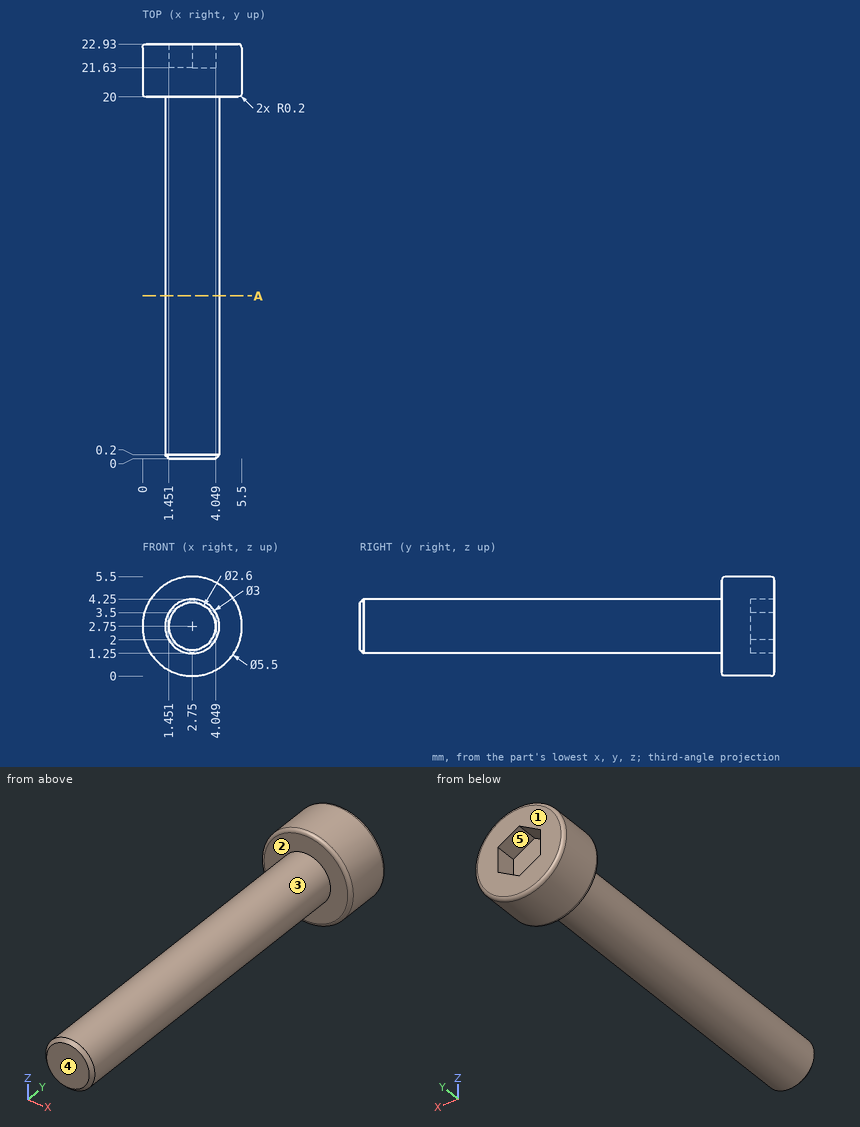
Verification items for this drawing (mm, ordinates from the low corner). A direction names the side the tool comes from. Round coordinates to 2 decimals unless told otherwise and drop trailing zeros. Order: outer loops, then holes, each group sorted by start corner. A loop starts at its lowest first (then second) coordinate and runs counter-clockwise, first axis right, second up.
1) Cross-section at A-A, the plane y = 9. Record the cut outline in (x, z), plus the area to 3 significant figures.
Geometry says:
outline: circle Ø3 at (2.75, 2.75)
area: 7.07 mm2
2) Tool access check on the marked faces 1 and 2. Record the directions out of +Z, -Z, +X, -X, +Y, -Y that give a thin tool (end or side, any length) a straight path to the whole face; none if there is none.
Geometry says:
face 1: +Z, -Z, +X, -X, +Y
face 2: -Y
3) Material ranges on line 1 (Y direction, x = 4.45, z = 1.4); line 2 (Y direction, x = 2.2, z = 2.1); line 3 (X direction, y = 14.5, z = 1.55), recorded low to high.
Geometry says:
line 1: y = 20 to 22.93
line 2: y = 0 to 21.63
line 3: x = 1.85 to 3.65
4) Depth check by flat-ended pin: pin 1 (1 mm diameter, centred on x = 4.5, y = 10, fed in from -Z); pin 2 (1.5 mm diameter, centred on y = 13.5, z = 4, fed in from -X). Enter the tip coordinate at first touch or a pass-through.
Geometry says:
pin 1: stops at z = 1.92
pin 2: stops at x = 1.34
5) Draft check along Z on the marked faces 3, 4 and 5. Enter one of: +Z half, -Z half, draft (parallel to the pull), parting line (faces both ways), or undercut.
Geometry says:
face 3: parting line
face 4: draft
face 5: undercut
